from build123d import *

# Parameters (mm, degrees)
SKIZZE6_W                       = 60
SKIZZE6_H                       = 23
AUFSATZ_LINEAR_AUSTRAGEN1_DEPTH = 4
SKIZZE7_R                       = 3.5
SCHNITT_LINEAR_AUSTRAGEN1_DEPTH = 5
VERRUNDUNG1_R                   = 10
SCHNITT_LINEAR_AUSTRAGEN2_DEPTH = 2
VERRUNDUNG2_R                   = 5
SCHNITT_LINEAR_AUSTRAGEN3_DEPTH = 5


with BuildPart() as part:
    # Skizze6 → Aufsatz-Linear austragen1 (new body)
    with BuildSketch(Plane.XY):
        with Locations((30, 6.5)):
            Rectangle(SKIZZE6_W, SKIZZE6_H)
    extrude(amount=AUFSATZ_LINEAR_AUSTRAGEN1_DEPTH)

    # Skizze7 → Schnitt-Linear austragen1 (cut, through all)
    with BuildSketch(Plane.XY.offset(4)):
        with Locations((6, 0)):
            Circle(SKIZZE7_R)
    extrude(amount=-SCHNITT_LINEAR_AUSTRAGEN1_DEPTH, mode=Mode.SUBTRACT)

    # Verrundung1
    verrundung1_edges = [part.edges().sort_by_distance(p)[0] for p in [
        (0, 18, 2),
        (60, 18, 2),
        (60, -5, 2),
    ]]
    fillet(verrundung1_edges, radius=VERRUNDUNG1_R)

    # Skizze9 → Schnitt-Linear austragen2 (cut)
    with BuildSketch(Plane.XY.offset(4)):
        with BuildLine():
            Line((6.281560008, 3.839690608), (22.131768578, 2.677413406))
            ThreePointArc((22.131768578, 2.677413406), (24.448770853, 0.212964842), (22.189275528, -2.304312884))
            Line((22.189275528, -2.304312884), (6.370120712, -3.83216788))
            ThreePointArc((6.370120712, -3.83216788), (2.150256489, -0.044439818), (6.281560008, 3.839690608))
        make_face()
    extrude(amount=-SCHNITT_LINEAR_AUSTRAGEN2_DEPTH, mode=Mode.SUBTRACT)

    # Verrundung2
    verrundung2_edges = [part.edges().sort_by_distance(p)[0] for p in [
        (0, -5, 2),
    ]]
    fillet(verrundung2_edges, radius=VERRUNDUNG2_R)

    # Skizze10 → Schnitt-Linear austragen3 (cut, through all)
    with BuildSketch(Plane.XY.offset(4)):
        with BuildLine():
            Line((18, 18), (0, 18))
            Line((0, 18), (0, 0))
            ThreePointArc((0, 0), (5.272077939, 12.727922061), (18, 18))
        make_face()
    extrude(amount=-SCHNITT_LINEAR_AUSTRAGEN3_DEPTH, mode=Mode.SUBTRACT)


solid = part.part
Model file for the job. Use its own axes, mm. A direction names the side the tool comes from. Coordinates: 2 decimals unless noted, no trailing zeros. Loops run counter-clockwise (first coordinate to the right, second up) from the corner with the lowest first, then second, coordinate; pieces in that order, holes last. Notation, with made-up numbers: (74.5, 16.25) -> (109.5, 16.25) arc R32 cw to (109.5, 54.25) -> close; hole circle Ø11 at (76, 63.5). An arc over 180 degrees is marked (long way). Use one line per item in the form item = value. Start each with the question number.
(1) Cut at D-D on y = -1.75. Give the cut face in (x, z), and give its area (3 significant figures).
(2) Flat gauge pins, fed straight in: pin 1 (1.5 mm diameter, centred on y = 2, z = 2, fed in from +X); pin 2 (6.5 mm diameter, centred on x = 6, y = 0, fed in from -Z). Where does each tip first touch, or does it go through?
(3) Pull direction X, two halves, no side cores. Call faces 3 (the flat face through (34, 18, 2)), 4 (the flat face through (14.39, -3.058, 3.014)), 5 (the cylindrical face through (5.133, 12.587, 2.028)): pulls with the +X half, pulls with the -X half, needs draft (parallel to the pull), parting line crosses it, or undercut.
(4) Cut at B-B on y = 1.75. Give the cut face in (x, z), and give its area (3 significant figures).
(5) Probe probe 1 along X at (y, z) = (0, 2.6); probe 2 along Y at (x, z) = (6, 2.5); probe 3 along Y at (x, z) = (11.5, 3.05). List the from-to ranges inside material, lowest first. Write a range as from..to.
(6) Cut at A-A on z = 0.8. Give the cut face in (x, y), and give its area (3 significant figures).
(7) Tool access for faces 1 (the flat face through (14.096, 3.267, 3.014)), 2 (the cylindrical face through (56.99, 15.15, 2.03)): list every direction of +Z, -Z, +X, -X, +Y, -Y with a clear straight run to the whole face (end or side of a thin tool).
(8) Cut at C-C on x = 14. Give the cut face in (y, z), and give its area (3 significant figures).
Values:
q1.outline = (0.32, 0) -> (2.97, 0) -> (2.97, 2) -> (2.57, 2) -> (2.57, 4) -> (0.32, 4) -> close; (9.03, 0) -> (57.38, 0) -> (57.38, 4) -> (23.53, 4) -> (23.53, 2) -> (9.03, 2) -> close
q1.area = 174 mm2
q2.pin_1 = 59.74
q2.pin_2 = through
q3.face_3 = needs draft
q3.face_4 = undercut
q3.face_5 = pulls with the -X half
q4.outline = (0.09, 0) -> (2.97, 0) -> (2.97, 2) -> (2.57, 2) -> (2.57, 4) -> (0.09, 4) -> close; (9.03, 0) -> (59.46, 0) -> (59.46, 4) -> (23.9, 4) -> (23.9, 2) -> (9.03, 2) -> close
q4.area = 183 mm2
q5.probe_1 = 0..2.15, 24.44..58.66
q5.probe_2 = -5..-3.85, 3.85..13.42
q5.probe_3 = -5..-3.34, 3.46..16.79
q6.outline = (0, 0) arc R5 ccw to (5, -5) -> (50, -5) arc R10 ccw to (60, 5) -> (60, 8) arc R10 ccw to (50, 18) -> (18, 18) arc R18 ccw to start; hole circle Ø7 at (6, 0)
q6.area = 1,220 mm2
q7.face_1 = +Z
q7.face_2 = +Z, -Z, +X, +Y
q8.outline = (-5, 0) -> (17.55, 0) -> (17.55, 4) -> (3.27, 4) -> (3.27, 2) -> (-3.1, 2) -> (-3.1, 4) -> (-5, 4) -> close
q8.area = 77.5 mm2
